Read the model definition and answer for the solid it produces. Units are mm, in the model's axes. A direction names the side the tool comes from. Coordinates: 2 decimals unless noted, no trailing zeros. Write each loop counter-clockwise with the first axis right and the second up, starting at its lowest first coordinate (ties: lowest second). Pieces come first, ordered by that corner, then holes. Notation, with made-up numbers: (49.5, 63.5) -> (75.5, 63.5) arc R28 ccw to (75.5, 94.5) -> close; hole circle Ø3 at (85.25, -18). An arc over 180 degrees is marked (long way). Answer in a Markdown table with one row per item. Add a question column.
Item 1: Section B-B on x = 55 is taken. Write down the section's boundary in (y, z), then the cut area to 3 significant figures.
Item 2: Straight lines are drawn through the part: line 1 (Y direction, x = 17, z = 13.15) (3 decimals); line 2 (Y direction, x = -17, z = 4.5); line 3 (X direction, y = -18, z = 3). For each, find the intervals that lie inside material, in ascending order. Write a range as from..to.
Item 3: Section C-C on z = 2 is taken. Write down the section's boundary in (x, y).
Item 4: Which of the six approach directions +Z, -Z, +X, -X, +Y, -Y give full straight-line access (tool end or side, diameter ignored) to faces 4 (the face through (13.96, 19.79, 13.03)), 5 (the face through (14.968, -17.843, 5.423))?
Item 5: Section A-A on x = -17 is taken. Write down the section's boundary in (y, z) (3 decimals).
Item 6: Given pin 1 Ø4 at (x, y) = (-17.5, -17.5) entering from +Z, flat-ended and moving along its own axis, determine where the tip first touches the part or whether it passes through.
Item 7: Section D-D on y = 17 is taken. Write down the section's boundary in (x, z) (3 decimals), then the cut area to 3 significant figures.
Item 8: For a pull along Y with two mould halves and no side action, classify faces 1 (the face through (-75, -1, 7)), 2 (the face through (-20.04, 19.79, 13.03)), 3 (the face through (-1, 58.75, 7)) as +Y half, -Y half, draft (parallel to the pull), parting line (faces both ways), or undercut.
```python
from build123d import *

# Parameters (mm, degrees)
F0_W           = 150
F0_H           = 117.5
F1_DEPTH       = 15
F3_D           = 10
F5_D           = 4.4
F5_CBORE_D     = 8.25
F5_CBORE_DEPTH = 4


with BuildPart() as f1:
    # F0 (on Top) → F1 (new body)
    with BuildSketch(Plane.XY):
        Rectangle(F0_W, F0_H)
    extrude(amount=F1_DEPTH)

    # F3 (through all)
    with Locations(Plane.XY.offset(15)):
        with Locations((-61, 17), (-61, -17), (55, 0)):
            Hole(F3_D / 2)

    # F5 (through all)
    with Locations(Plane.XY.offset(15)):
        with Locations((-17, 17), (17, 17), (17, -17), (-17, -17)):
            CounterBoreHole(F5_D / 2, F5_CBORE_D / 2, F5_CBORE_DEPTH)


solid = f1.part
```
Results below:
| question | item | result |
|---|---|---|
| 1 | outline | (-58.75, 0) -> (-5, 0) -> (-5, 15) -> (-58.75, 15) -> close; (5, 0) -> (58.75, 0) -> (58.75, 15) -> (5, 15) -> close |
| 1 | area | 1,610 mm2 |
| 2 | line 1 | y = -58.75..-21.125, -12.875..12.875, 21.125..58.75 |
| 2 | line 2 | y = -58.75..-19.2, -14.8..14.8, 19.2..58.75 |
| 2 | line 3 | x = -75..-65.9, -56.1..-18.96, -15.04..15.04, 18.96..75 |
| 3 | outline | (-75, -58.75) -> (75, -58.75) -> (75, 58.75) -> (-75, 58.75) -> close; hole circle Ø10 at (-61, -17); hole circle Ø10 at (-61, 17); hole circle Ø4.4 at (-17, -17); hole circle Ø4.4 at (-17, 17); hole circle Ø4.4 at (17, -17); hole circle Ø4.4 at (17, 17); hole circle Ø10 at (55, 0) |
| 4 | face 4 | +Z |
| 4 | face 5 | +Z, -Z |
| 5 | outline | (-58.75, 0) -> (-19.2, 0) -> (-19.2, 11) -> (-21.125, 11) -> (-21.125, 15) -> (-58.75, 15) -> close; (-14.8, 0) -> (14.8, 0) -> (14.8, 11) -> (12.875, 11) -> (12.875, 15) -> (-12.875, 15) -> (-12.875, 11) -> (-14.8, 11) -> close; (19.2, 0) -> (58.75, 0) -> (58.75, 15) -> (21.125, 15) -> (21.125, 11) -> (19.2, 11) -> close |
| 6 | pin 1 | stops at z = 11 |
| 7 | outline | (-75, 0) -> (-66, 0) -> (-66, 15) -> (-75, 15) -> close; (-56, 0) -> (-19.2, 0) -> (-19.2, 11) -> (-21.125, 11) -> (-21.125, 15) -> (-56, 15) -> close; (-14.8, 0) -> (14.8, 0) -> (14.8, 11) -> (12.875, 11) -> (12.875, 15) -> (-12.875, 15) -> (-12.875, 11) -> (-14.8, 11) -> close; (19.2, 0) -> (75, 0) -> (75, 15) -> (21.125, 15) -> (21.125, 11) -> (19.2, 11) -> close |
| 7 | area | 1,940 mm2 |
| 8 | face 1 | draft |
| 8 | face 2 | undercut |
| 8 | face 3 | +Y half |
